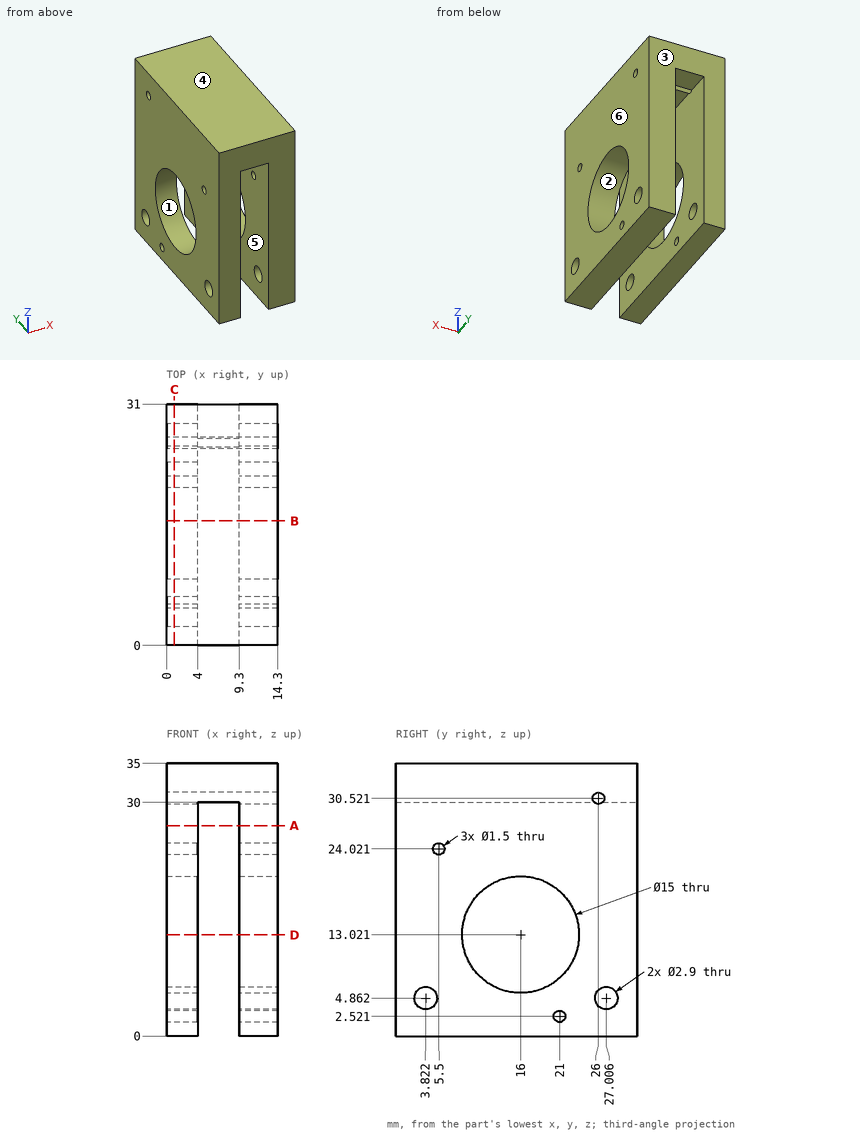
Drawing for the job (mm, zero at the part's lowest x, y, z). A direction names the side the tool comes from. Give positions to 0.01 mm unless a question says otherwise; leave off trailing zeros. Order: outer loops, then holes, each group sorted by start corner. A loop starts at its lowest first (then second) coordinate and runs counter-clockwise, first axis right, second up. Notation, with made-up numbers: M -34,-6.75 L -18,-6.75 A21 cw -18,5.25 Z; hole C -9.75,-23 d2. An arc over 180 degrees is marked long. Write item = value, one per line. Start each with the question number.
(1) Slice it at B-B on y = 16. Write the cut outline in (x, z).
(2) Slice it at D-D on z = 13. Write the cut outline in (x, y).
(3) Slice it at C-C on x = 1. Write the cut outline in (y, z), plus the area to 3 significant figures.
(4) Slice it at A-A on z = 27. Write the cut outline in (x, y).
(5) Pin check, flat tip, straight feed: pin 1 Ø1.3 at (x, y) = (6.5, 29.5) entering from -Z. Stop position of the tip, or through.
(6) Two-plate mould, pull along Z, no slides. Class the marked faces 1, 2, 3 and 4: released by +Z, released by -Z, zero draft, split by the parting line, or undercut.
(7) Which spindle directions (+Z, -Z, +X, -X, +Y, -Y) get a long thin tool onto all of the face, cutting with end or side? Do the marked faces 5 and 6. Say none if no direction does.
(8) Probe L1, parallel to X at y = 18.5, z = 24; L2, parallel to Z at x = 10, y = 18; L3, parallel to Y at x = 11, z = 7. List the from-to ranges inside material, lowest first. Write a range as [from, to].
Responses:
q1.outline = M 0,0 L 4,0 L 4,5.52 L 0,5.52 Z; M 0,20.52 L 4,20.52 L 4,30 L 9.3,30 L 9.3,20.52 L 14.3,20.52 L 14.3,35 L 0,35 Z; M 9.3,0 L 14.3,0 L 14.3,5.52 L 9.3,5.52 Z
q2.outline = M 0,0 L 4,0 L 4,8.5 L 0,8.5 Z; M 0,23.5 L 4,23.5 L 4,31 L 0,31 Z; M 9.3,0 L 14.3,0 L 14.3,8.5 L 9.3,8.5 Z; M 9.3,23.5 L 14.3,23.5 L 14.3,31 L 9.3,31 Z
q3.outline = M 0,0 L 31,0 L 31,35 L 0,35 Z; hole C 3.82,4.86 d2.9; hole C 5.5,24.02 d1.5; hole C 16,13.02 d15; hole C 21,2.52 d1.5; hole C 26,30.52 d1.5; hole C 27.01,4.86 d2.9
q3.area = 890 mm2
q4.outline = M 0,0 L 4,0 L 4,31 L 0,31 Z; M 9.3,0 L 14.3,0 L 14.3,31 L 9.3,31 Z
q5.pin_1 = 30
q6.face_1 = undercut
q6.face_2 = undercut
q6.face_3 = zero draft
q6.face_4 = released by +Z
q7.face_5 = -Z, +Y, -Y
q7.face_6 = +Z, -Z, +X, +Y, -Y
q8.L1 = [0, 4], [9.3, 14.3]
q8.L2 = [0, 5.79], [20.25, 35]
q8.L3 = [0, 11.53], [20.47, 31]
